Input: part model. Units: mm. Frame: model coordinates. A direction names the side the tool comes from. Round coordinates to 2 decimals unless told otherwise and drop trailing zeros. Loops run counter-clockwise (first coordinate to the right, second up) from the corner with the lowest first, then second, coordinate; pieces in that order, holes last. Notation, with made-up numbers: (27.25, -14.5) -> (67.25, -14.5) arc R21 ccw to (67.25, -7.5) -> close; hole circle Ø8 at (74, 62.25). An arc over 180 degrees is marked (long way). Answer as a JSON object with one key per item and string values.
```python
from build123d import *

# Parameters (mm, degrees)
BOSS_EXTRUDE1_DEPTH        = 10
BOSS_EXTRUDE1_DEPTH_BACK   = 10
BOSS_EXTRUDE1_2_DEPTH      = 10
BOSS_EXTRUDE1_2_DEPTH_BACK = 10
SKETCH1_R                  = 10
BOSS_EXTRUDE3_DEPTH        = 5
BOSS_EXTRUDE3_DEPTH_BACK   = 5


with BuildPart() as part:
    # Sketch1 → Boss-Extrude1 (new, two sides: drawn at the far end of the back side and taken through both)
    with BuildSketch(Plane.XY.offset(-BOSS_EXTRUDE1_DEPTH_BACK)):
        with BuildLine():
            ThreePointArc((-114.782571429, 28.360206209), (-130.845692202, -15.231552601), (-84.928968254, -22.296943393))
            ThreePointArc((-84.928968254, -22.296943393), (-77.594426184, -12.203873312), (-75, 0))
            ThreePointArc((-75, 0), (-75.083767584, 2.240320966), (-75.334602536, 4.468130848))
            ThreePointArc((-75.334602536, 4.468130848), (-76.92830233, 10.582050364), (-79.767134466, 16.226598441))
            ThreePointArc((-79.767134466, 16.226598441), (-95.177372737, 28.346357679), (-114.782571429, 28.360206209))
        make_face()
        with BuildLine():
            Line((-101, 18), (-101, 14.456832295))
            ThreePointArc((-101, 14.456832295), (-105, -15), (-109, 14.456832295))
            Line((-109, 14.456832295), (-109, 18))
            Line((-109, 18), (-101, 18))
        make_face(mode=Mode.SUBTRACT)
    extrude(amount=BOSS_EXTRUDE1_DEPTH + BOSS_EXTRUDE1_DEPTH_BACK)



with BuildPart() as body_2:
    # Sketch1 → Boss-Extrude1 2 (new, two sides: drawn at the far end of the back side and taken through both)
    with BuildSketch(Plane.XY.offset(-BOSS_EXTRUDE1_2_DEPTH_BACK)):
        with BuildLine():
            ThreePointArc((-19.846557236, 5.134604745), (-19.158178407, -7.294806381), (-11.40536084, -17.034310791))
            ThreePointArc((-11.40536084, -17.034310791), (9.655053153, -18.083969382), (20.5, 0))
            ThreePointArc((20.5, 0), (17.620554998, 10.476929014), (9.791117897, 18.010663795))
            ThreePointArc((9.791117897, 18.010663795), (-5.273160122, 19.810193899), (-17.449330151, 10.759687601))
            ThreePointArc((-17.449330151, 10.759687601), (-18.858849203, 8.037027232), (-19.846557236, 5.134604745))
        make_face()
        Circle(SKETCH1_R, mode=Mode.SUBTRACT)
    extrude(amount=BOSS_EXTRUDE1_2_DEPTH + BOSS_EXTRUDE1_2_DEPTH_BACK)


with BuildPart() as part_1:
    add(part.part)

    add(body_2.part)  # Boss-Extrude3 merges body 2
    # Sketch1_5 → Boss-Extrude3 (add, two sides: drawn at the far end of the back side and taken through both)
    with BuildSketch(Plane.XY.offset(-BOSS_EXTRUDE3_DEPTH_BACK)):
        with BuildLine():
            ThreePointArc((-17.449330151, 10.759687601), (-5.273160122, 19.810193899), (9.791117897, 18.010663795))
            ThreePointArc((9.791117897, 18.010663795), (-51.406147601, 36.300304325), (-114.782571429, 28.360206209))
            ThreePointArc((-114.782571429, 28.360206209), (-95.177372737, 28.346357679), (-79.767134466, 16.226598441))
            ThreePointArc((-79.767134466, 16.226598441), (-80.178220113, 24.162367707), (-73.54479246, 28.537646307))
            ThreePointArc((-73.54479246, 28.537646307), (-47.487956655, 27.874909654), (-21.957791125, 22.620524811))
            ThreePointArc((-21.957791125, 22.620524811), (-16.78083736, 17.80107195), (-17.449330151, 10.759687601))
        make_face()
        with BuildLine():
            ThreePointArc((-84.928968254, -22.296943393), (-49.070592623, -7.043942052), (-11.40536084, -17.034310791))
            ThreePointArc((-11.40536084, -17.034310791), (-19.158178407, -7.294806381), (-19.846557236, 5.134604745))
            ThreePointArc((-19.846557236, 5.134604745), (-23.446258475, 0.296093427), (-29.401591979, -0.654192653))
            ThreePointArc((-29.401591979, -0.654192653), (-47.309577117, 1.062360507), (-65.040995656, -1.977258391))
            ThreePointArc((-65.040995656, -1.977258391), (-71.669449556, -1.120833178), (-75.334602536, 4.468130848))
            ThreePointArc((-75.334602536, 4.468130848), (-75.083767584, 2.240320966), (-75, 0))
            ThreePointArc((-75, 0), (-77.594426184, -12.203873312), (-84.928968254, -22.296943393))
        make_face()
    extrude(amount=BOSS_EXTRUDE3_DEPTH + BOSS_EXTRUDE3_DEPTH_BACK)


solid = part_1.part
```
1) Reachability of faces 5 (the face through (-71.59, -1.17, -0.07)), 6 (the face through (-5, -9, 10)) from +Z, -Z, +X, -X, +Y, -Y: full face, straight path, thin tool, end or side. Return the list, or none.
Output:
{"face 5": "+Z, -Z", "face 6": "+Z, +X, -X, +Y, -Y"}
2) Section A-A, the plane z = 7. Output: boundary loops of the cut face in (x, y), plus the area to 3 significant figures.
Output:
{"outline": "circle Ø60 at (-105, 0); circle Ø41 at (0, 0); hole (-109, 14.46) arc R15 ccw (long way) to (-101, 14.46) -> (-101, 18) -> (-109, 18) -> close; hole circle Ø20 at (0, 0)", "area": "3,100 mm^2"}
3) Section B-B, the plane x = -105. Output: boundary loops of the cut face in (y, z).
Output:
{"outline": "(-30, -10) -> (-15, -10) -> (-15, 10) -> (-30, 10) -> close; (18, -10) -> (30, -10) -> (30, -5) -> (31.38, -5) -> (31.38, 5) -> (30, 5) -> (30, 10) -> (18, 10) -> close"}
4) Draft query along Y for faces 1 (the face through (-49.625, -7.086, -0.07)), 2 (the face through (-101, 16, 0)), 3 (the face through (-53, 29, 5)), 4 (the face through (-50.509, 36.223, -0.07)). Return one class per face: +Y half, -Y half, draft (parallel to the pull), parting line (faces both ways), or undercut.
Output:
{"face 1": "-Y half", "face 2": "undercut", "face 3": "draft", "face 4": "+Y half"}
5) Section C-C, the plane z = -2.75. Output: boundary loops of the cut face in (x, y), plus the area to 3 significant figures.
Output:
{"outline": "(-114.78, 28.36) arc R30 ccw (long way) to (-84.93, -22.3) arc R60 cw to (-11.41, -17.03) arc R20.5 ccw (long way) to (9.79, 18.01) arc R155 ccw to start; hole (-109, 14.46) arc R15 ccw (long way) to (-101, 14.46) -> (-101, 18) -> (-109, 18) -> close; hole (-79.77, 16.23) arc R30 cw to (-75.33, 4.47) arc R8 ccw to (-65.04, -1.98) arc R68 cw to (-29.4, -0.65) arc R8 ccw to (-19.85, 5.13) arc R20.5 cw to (-17.45, 10.76) arc R8 ccw to (-21.96, 22.62) arc R147 ccw to (-73.54, 28.54) arc R8 ccw to start; hole circle Ø20 at (0, 0)", "area": "4,520 mm^2"}
6) Ray query, probe 1 along X at (y, z) = (8.5, 8.5); probe 2 along X at (y, z) = (16.5, -2.25); probe 3 along X at (y, z) = (-1, 8.75). Return the intervals inside material, ascending.
Output:
{"probe 1": "x = -133.77 to -117.36, -92.64 to -76.23, -18.65 to -5.27, 5.27 to 18.65", "probe 2": "x = -130.05 to -109, -101 to -79.94, -16.41 to 12.17", "probe 3": "x = -134.98 to -119.97, -90.03 to -75.02, -20.48 to -9.95, 9.95 to 20.48"}
7) Section D-D, the plane x = 0. Output: boundary loops of the cut face in (y, z).
Output:
{"outline": "(-20.5, -10) -> (-10, -10) -> (-10, 10) -> (-20.5, 10) -> close; (10, -10) -> (20.5, -10) -> (20.5, -5) -> (22.89, -5) -> (22.89, 5) -> (20.5, 5) -> (20.5, 10) -> (10, 10) -> close"}
8) Contact query for flat-ended pins moving along their axis: P1, Ø1, axis at y = 10, z = 6.5, coming from the -X side; P2, Ø13.5, axis at x = -43, y = -13, coming from the -Z side; P3, Ø12, axis at x = -1.5, z = 7.5, coming from the -Y side. Output: stop coordinate, or through.
Output:
{"P1": "stops at x = -133.46", "P2": "stops at z = -5", "P3": "stops at y = -20.5"}
